```python
from build123d import *

# Parameters (mm, degrees)
BOSS_EXTRUDE1_DEPTH = 10
SKETCH2_R           = 1.5
CUT_EXTRUDE1_DEPTH  = 5


with BuildPart() as part:
    # Sketch1 → Boss-Extrude1 (new body)
    with BuildSketch(Plane.XY):
        with BuildLine():
            Line((20, 0), (20, -320))
            Line((20, -320), (17, -320))
            Line((17, -320), (17, 0))
            ThreePointArc((17, 0), (12.02081528, 12.02081528), (0, 17))
            Line((0, 17), (-60, 17))
            Line((-60, 17), (-60, 20))
            Line((-60, 20), (0, 20))
            ThreePointArc((0, 20), (14.142135624, 14.142135624), (20, 0))
        make_face()
    extrude(amount=BOSS_EXTRUDE1_DEPTH)

    # Sketch2 → Cut-Extrude1 (cut)
    with BuildSketch(Plane(origin=(0, 20, 0), x_dir=(1, 0, 0), z_dir=(0, 1, 0))):
        with Locations(Location((-54.5, -5, 0), (0, 0, 180))):
            Circle(SKETCH2_R)
    extrude(amount=-CUT_EXTRUDE1_DEPTH, mode=Mode.SUBTRACT)


solid = part.part
```
Could you check a few things on this model? Use its own coordinates, in mm. A direction names the side the tool comes from. Give positions to 0.01 mm unless a question says otherwise; leave off trailing zeros. Loops run counter-clockwise (first coordinate to the right, second up) from the corner with the lowest first, then second, coordinate; pieces in that order, holes last. Notation, with made-up numbers: (-14, -16) - (38, -16) arc R30 cw to (38, 14) - close; hole circle Ø7 at (-20, -13). An arc over 180 degrees is marked (long way). Answer in a Markdown table with one row per item. Add a question column.
Q1. Please list where these lines run through material, in increasing order: L1, parallel to Z at x = -54.5, y = 19.35; L2, parallel to X at y = -79.5, z = 1.5. Write a range as from..to.
Q2. For pin 1 (12 mm diameter, centred on x = 9.5, y = -59.5, fed in from +Z); pin 2 (1 mm diameter, centred on y = -222.5, z = 4, fed in from -X); pin 3 (5 mm diameter, centred on x = -29, z = 4.5, fed in from -Y), each with a flat end and sliding along its axis, tell me the tip position at first contact or that it passes through.
Q3. If we section it at B-B (y = -117.5): List the corners of the cut face in (x, z) for me.
Q4. If we section it at A-A (z = 5): List the corners of the cut face in (x, y) for me.
Q5. Which directions (+Z, -Z, +X, -X, +Y, -Y) give clear straight access to the entire face, cutting with the end or side of a thin tool? Please do faces 1 (the face through (17, -162, 5)), 2 (the face through (19, -149, 0)).
The answers:
| question | item | result |
|---|---|---|
| 1 | L1 | z = 0..3.5, 6.5..10 |
| 1 | L2 | x = 17..20 |
| 2 | pin 1 | passes through |
| 2 | pin 2 | stops at x = 17 |
| 2 | pin 3 | stops at y = 17 |
| 3 | outline | (17, 0) - (20, 0) - (20, 10) - (17, 10) - close |
| 4 | outline | (-60, 17) - (-56, 17) - (-56, 20) - (-60, 20) - close; (-53, 17) - (0, 17) arc R17 cw to (17, 0) - (17, -320) - (20, -320) - (20, 0) arc R20 ccw to (0, 20) - (-53, 20) - close |
| 5 | face 1 | +Z, -Z, -X, -Y |
| 5 | face 2 | -Z, +X, -X, +Y, -Y |
